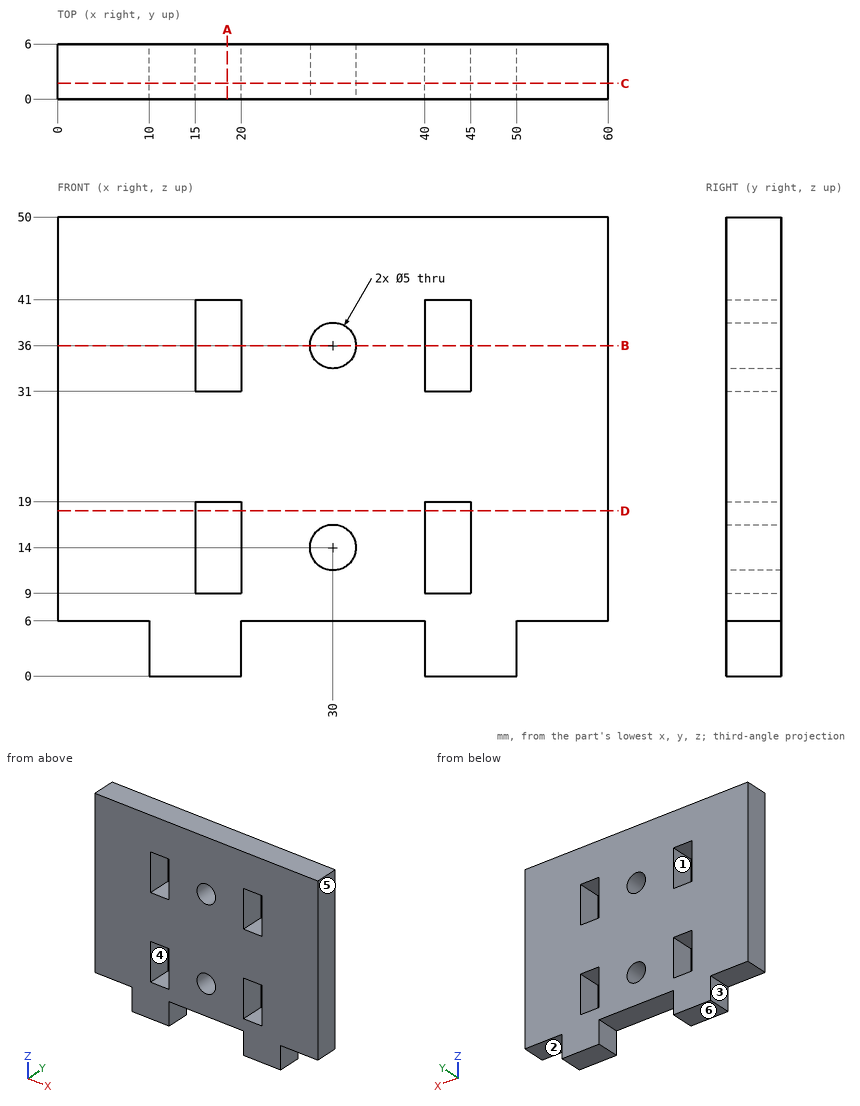
Can you work these out from the drawing? Everything is in mm from the part's minimum corner. A direction names the side the tool comes from. Round coordinates to 2 decimals unless told otherwise and drop trailing zeros. Loops run counter-clockwise (first coordinate to the right, second up) from the corner with the lowest first, then second, coordinate; pieces in that order, holes last. Notation, with made-up numbers: (37.5, -24) - (78.5, -24) arc R21 cw to (78.5, -1) - close; hole circle Ø4 at (-32, -1). An arc over 180 degrees is marked (long way). Answer in a Markdown table with one row per item. Add a question column.
Q1. Which directions (+Z, -Z, +X, -X, +Y, -Y) give clear straight access to the entire face, cutting with the end or side of a thin tool? Please do the marked faces 1, 2 and 3.
Q2. We'd pull the mould along Z, two halves only. Please class the marked faces 4, 5 and 6: pulls with the +Z half, pulls with the -Z half, needs draft (parallel to the pull), parting line crosses it, or undercut.
Q3. I want a section at B-B on z = 36. List the corners of the cut face in (x, y) for me.
Q4. For pin 1 Ø3 at (x, y) = (3.5, 3.5) entering from -Z; pin 2 Ø1.8 at (y, z) = (4.5, 2) entering from -X, each with a flat end and sliding along its axis, tell me the tip position at first contact or that it passes through.
Q5. I want a section at C-C on y = 1.7. Count the separate pieces of the cut face and the enclosed holes in it, and give its area (3 significant figures).
Q6. I want a section at D-D on z = 18. List the corners of the cut face in (x, y) for me, and give its area (3 significant figures).
Q7. I want a section at A-A on x = 18.5. List the corners of the cut face in (y, z) for me, and give its area (3 significant figures).
Q8. I need wall thicknesses on L1, parallel to X at y = 4.2, z = 36; L2, parallel to X at y = 1.7, z = 33; L3, parallel to Z at x = 29.5, y = 4.95. Which ranges of each line are inside material? Lowest first, please.
A:
| question | item | result |
|---|---|---|
| 1 | face 1 | +Y, -Y |
| 1 | face 2 | -Z, +X, +Y, -Y |
| 1 | face 3 | -Z, -X, +Y, -Y |
| 2 | face 4 | undercut |
| 2 | face 5 | needs draft |
| 2 | face 6 | pulls with the -Z half |
| 3 | outline | (0, 0) - (15, 0) - (15, 6) - (0, 6) - close; (20, 0) - (27.5, 0) - (27.5, 6) - (20, 6) - close; (32.5, 0) - (40, 0) - (40, 6) - (32.5, 6) - close; (45, 0) - (60, 0) - (60, 6) - (45, 6) - close |
| 4 | pin 1 | z = 6 |
| 4 | pin 2 | x = 10 |
| 5 | separate pieces | 1 |
| 5 | enclosed holes | 6 |
| 5 | area | 2,520 mm^2 |
| 6 | outline | (0, 0) - (15, 0) - (15, 6) - (0, 6) - close; (20, 0) - (40, 0) - (40, 6) - (20, 6) - close; (45, 0) - (60, 0) - (60, 6) - (45, 6) - close |
| 6 | area | 300 mm^2 |
| 7 | outline | (0, 0) - (6, 0) - (6, 9) - (0, 9) - close; (0, 19) - (6, 19) - (6, 31) - (0, 31) - close; (0, 41) - (6, 41) - (6, 50) - (0, 50) - close |
| 7 | area | 180 mm^2 |
| 8 | L1 | 0 to 15, 20 to 27.5, 32.5 to 40, 45 to 60 |
| 8 | L2 | 0 to 15, 20 to 40, 45 to 60 |
| 8 | L3 | 6 to 11.55, 16.45 to 33.55, 38.45 to 50 |
